Geometry check sheet. Reference: the model listing, model coordinates, mm. Face numbers are marked on the shaded views. Round coordinates to 2 decimals unless told otherwise and drop trailing zeros. Order: outer loops, then holes, each group sorted by start corner. A loop starts at its lowest first (then second) coordinate and runs counter-clockwise, first axis right, second up.
```python
from build123d import *

# Parameters (mm, degrees)
SKETCH1_W           = 5
SKETCH1_H           = 1
BOSS_EXTRUDE1_DEPTH = 1
SKETCH3_R           = 1
BOSS_EXTRUDE2_DEPTH = 5


with BuildPart() as part:
    # Sketch1 → Revolve1 (revolve)
    with BuildSketch(Plane(origin=(0, 0, 0), x_dir=(1, 0, 0), z_dir=(0, 1, 0))):
        with Locations((32.5, 0.5)):
            Rectangle(SKETCH1_W, SKETCH1_H)
    revolve(axis=Axis((0, 0, 0), (0, 0, -1)))

    # Sketch2 → Boss-Extrude1 (add)
    with BuildSketch(Plane(origin=(0, 0, -1), x_dir=(-1, 0, 0), z_dir=(0, 0, -1))):
        Polygon((-2, -30.927225956), (2, -30.927225956), (2, -2), (31.252775703, -2), (31.252775703, 2), (2, 2), (2, 30.927225956), (-2, 30.927225956), (-2, 2), (-31.252775703, 2), (-31.252775703, -2), (-2, -2), align=None)
    extrude(amount=-BOSS_EXTRUDE1_DEPTH)

    # Sketch3 → Boss-Extrude2 (add)
    with BuildSketch(Plane(origin=(0, 0, -1), x_dir=(-1, 0, 0), z_dir=(0, 0, -1))):
        with Locations((-32.071898489, 0)):
            Circle(SKETCH3_R)
        with Locations(Location((32.071898489, 0, 0), (0, 0, 180))):
            Circle(SKETCH3_R)
    extrude(amount=BOSS_EXTRUDE2_DEPTH)


solid = part.part
```
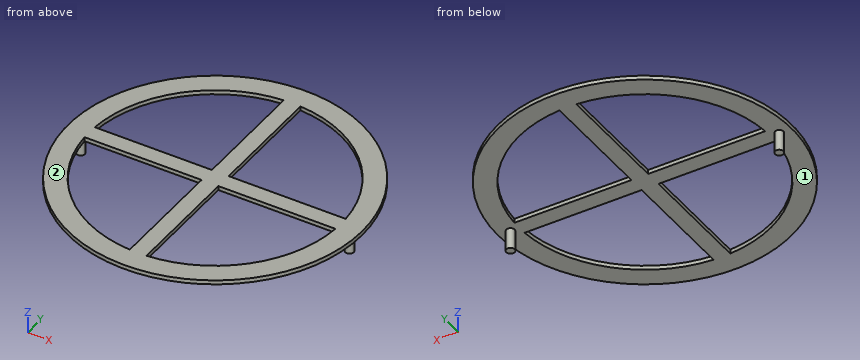
(1) Sectioned sample at A-A, the plane x = -8. Record the cut outline in (y, z).
Returned:
outline: (-34.07, -1) - (-28.91, -1) - (-28.91, 0) - (-34.07, 0) - close; (-2, -1) - (2, -1) - (2, 0) - (-2, 0) - close; (28.91, -1) - (34.07, -1) - (34.07, 0) - (28.91, 0) - close
(2) Draft check along X on the marked faces 1 and 2. Enter one of: released by +X, released by -X, zero draft, split by the parting line, or undercut.
Returned:
face 1: undercut
face 2: zero draft
(3) Material ranges on line 1 (Y direction, x = 3, z = -0.6); line 2 (Z direction, x = -12, y = -31); line 3 (Y direction, x = -14, z = -0.75), recorded low to high.
Returned:
line 1: y = -34.87 to -29.85, -2 to 2, 29.85 to 34.87
line 2: z = -1 to 0
line 3: y = -32.08 to -26.53, -2 to 2, 26.53 to 32.08
(4) Sectioned sample at B-B, the plane y = -19.5. Record the cut outline in (x, z), and give its area (3 significant figures).
Returned:
outline: (-29.06, -1) - (-22.8, -1) - (-22.8, 0) - (-29.06, 0) - close; (-2, -1) - (2, -1) - (2, 0) - (-2, 0) - close; (22.8, -1) - (29.06, -1) - (29.06, 0) - (22.8, 0) - close
area: 16.5 mm2
(5) Depth check by flat-ended pin: P1, Ø1.1, axis at y = 18, z = -0.5, coming from the +X side; P2, Ø1, axis at x = 27.5, z = -1, coming from the +Y side; P3, Ø3, axis at x = -9.5, z = -1, coming from the +Y side; P4, Ø5, axis at x = -6, y = -24.5, coming from the +Z side. Enter the tip coordinate at first touch or a pass-through.
Returned:
P1: stops at x = 30.34
P2: stops at y = 22.27
P3: stops at y = 34.07
P4: passes through
